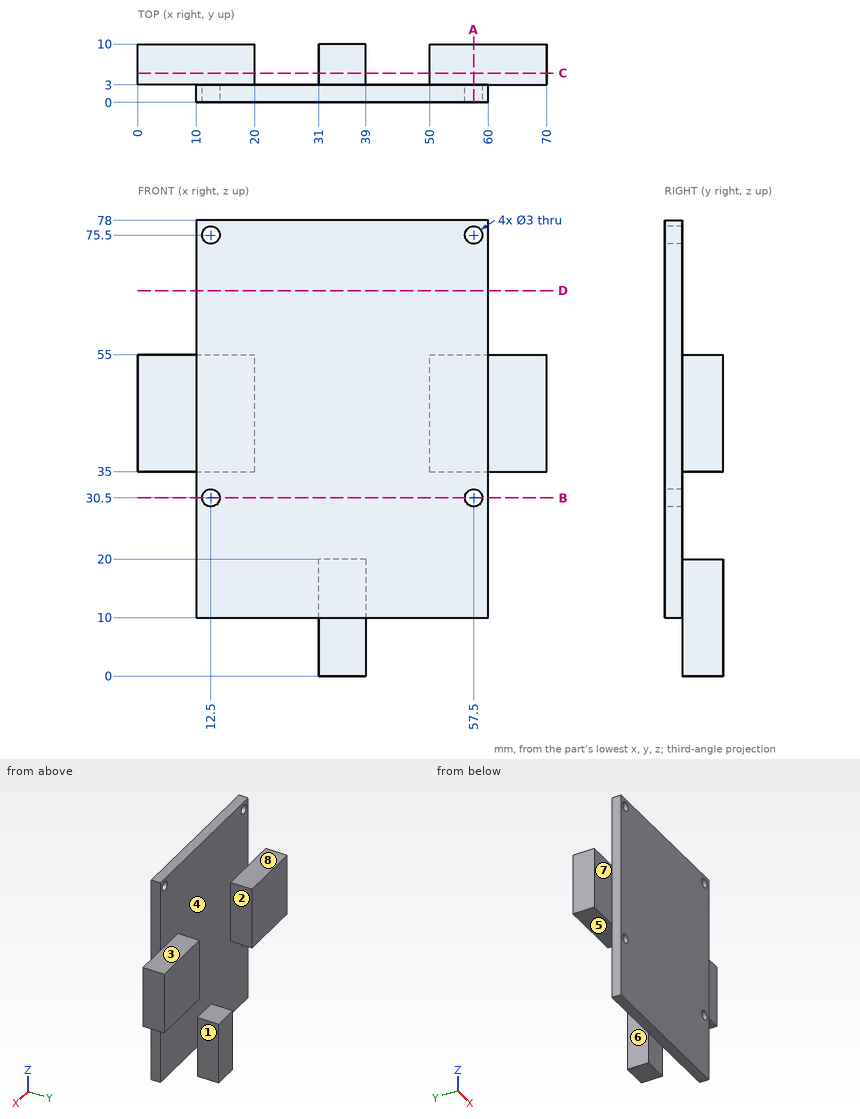
The drawing under review shows one solid part. Ordinate dimensions are in mm from its lowest x, y, z. A direction names the side the tool comes from. Give positions to 0.01 mm unless a question says otherwise; leave off trailing zeros. Order: outer loops, then holes, each group sorted by start corner. A loop starts at its lowest first (then second) coordinate and runs counter-clockwise, first axis right, second up. Notation, with made-up numbers: M 81.25,-37.5 L 105.25,-37.5 A24 cw 105.25,-4.5 Z; hole C 17.5,46 d9. An arc over 180 degrees is marked long. Answer in a Markdown table with one row per item. Add a question column.
1. Add section B-B on z = 30.5. State the section outline as (x, y) points.
2. Machinability: for the marked faces 5, 6, 7 and 8, which of the approach directions +Z, -Z, +X, -X, +Y, -Y give a long, thin tool a straight path to every point of the face, cutting with its end or side? Answer none if there is none.
3. Add section D-D on z = 66. State the section outline as (x, y) points, plus the area to 3 significant figures.
4. For pin 1 Ø1.5 at (x, y) = (23.5, 2) entering from -Z; pin 2 Ø3.5 at (y, z) = (1, 59) entering from +X; pin 3 Ø2 at (x, y) = (13.5, 8) entering from +Z; pin 4 Ø6 at (x, y) = (45.5, 8.5) entering from -Z, all flat-tipped, find the tip position at first contact; note any pin that passes through.
5. Add section C-C on y = 5. State the section outline as (x, z) points.
6. Mouldability with a two-part tool opening along X and no side actions: class the marked faces 1, 2, 3 and 4 as released by +X, released by -X, zero draft, split by the parting line, or undercut.
7. To check wall thickness, follow line 1 along Z through (x, y) = (57.5, 2.35); line 2 along X through (y, z) = (2.3, 75.5); line 3 along X through (y, z) = (5.75, 46). State the ranges of each line that lie inside material, in increasing order.
8. Add section A-A on x = 57.5. State the section outline as (y, z) points, plus the area to 3 significant figures.
The answers:
| question | item | result |
|---|---|---|
| 1 | outline | M 10,0 L 11,0 L 11,3 L 10,3 Z; M 14,0 L 56,0 L 56,3 L 14,3 Z; M 59,0 L 60,0 L 60,3 L 59,3 Z |
| 2 | face 5 | -Z, +X, -X, +Y |
| 2 | face 6 | +Z, -Z, -X, +Y |
| 2 | face 7 | +Z, -Z, -X, -Y |
| 2 | face 8 | +Z, +X, -X, +Y |
| 3 | outline | M 10,0 L 60,0 L 60,3 L 10,3 Z |
| 3 | area | 150 mm2 |
| 4 | pin 1 | z = 10 |
| 4 | pin 2 | x = 60 |
| 4 | pin 3 | z = 55 |
| 4 | pin 4 | through |
| 5 | outline | M 0,35 L 20,35 L 20,55 L 0,55 Z; M 31,0 L 39,0 L 39,20 L 31,20 Z; M 50,35 L 70,35 L 70,55 L 50,55 Z |
| 6 | face 1 | released by +X |
| 6 | face 2 | undercut |
| 6 | face 3 | zero draft |
| 6 | face 4 | undercut |
| 7 | line 1 | 10 to 29, 32 to 74, 77 to 78 |
| 7 | line 2 | 10 to 11, 14 to 56, 59 to 60 |
| 7 | line 3 | 0 to 20, 50 to 70 |
| 8 | outline | M 0,10 L 3,10 L 3,29 L 0,29 Z; M 0,32 L 3,32 L 3,35 L 10,35 L 10,55 L 3,55 L 3,74 L 0,74 Z; M 0,77 L 3,77 L 3,78 L 0,78 Z |
| 8 | area | 326 mm2 |
